Here's the drawing with two shaded views (mm, measured from the low corner). I have some questions. Give positions to 0.01 mm unless a question says otherwise; leave off trailing zeros. Loops run counter-clockwise (first coordinate to the right, second up) from the corner with the lowest first, then second, coordinate; pieces in that order, holes last. Notation, with made-up numbers: M 75.25,20 L 95.25,20 A21 ccw 95.25,39 Z; hole C 23,1.25 d8. An arc over 180 degrees is marked long. Put each result on its own line as item: value. Start each with the question number.
1) Please list where these lines run through material, in increasing order: line 1 along X through (y, z) = (25, 2.35); line 2 along Y through (x, z) = (63, 1); line 3 along X through (y, z) = (11, 2.7). Write a range as from..to.
2) Imagine slicing it at D-D (x = 92). Write out the boundary of the cut face in (y, z).
3) Imagine slicing it at C-C (z = 1). Write out the boundary of the cut face in (x, y), then the cut area to 3 significant figures.
4) Imagine slicing it at A-A (x = 57). Write out the boundary of the cut face in (y, z), then the cut area to 3 significant figures.
5) For P1, Ø1, axis at x = 22.5, y = 31.5, coming from the -Z side; P2, Ø1.5, axis at x = 50.5, z = 2, coming from the -Y side, each with a flat end and sliding along its axis, tell me the tip position at first contact or that it passes through.
6) Imagine slicing it at B-B (y = 5). Write out the boundary of the cut face in (x, z), then the cut area to 3 significant figures.
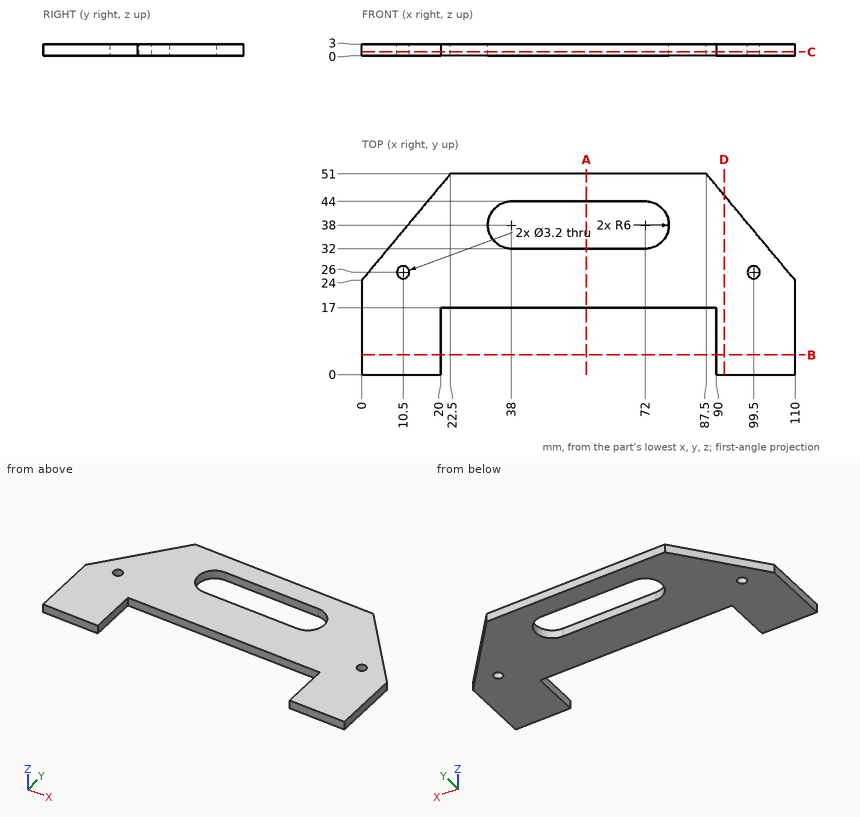
Recorded:
1. line 1: 0.83..9.25, 11.75..98.25, 100.75..109.17
1. line 2: 17..32, 44..51
1. line 3: 0..20, 90..110
2. outline: M 0,0 L 45.6,0 L 45.6,3 L 0,3 Z
3. outline: M 0,0 L 20,0 L 20,17 L 90,17 L 90,0 L 110,0 L 110,24 L 87.5,51 L 22.5,51 L 0,24 Z; hole C 10.5,26 d3.2; hole M 38,32 L 72,32 A6 ccw 72,44 L 38,44 A6 ccw Z; hole C 99.5,26 d3.2
3. area: 3,280 mm²
4. outline: M 17,0 L 32,0 L 32,3 L 17,3 Z; M 44,0 L 51,0 L 51,3 L 44,3 Z
4. area: 66.0 mm²
5. P1: z = 0
5. P2: y = 17
6. outline: M 0,0 L 20,0 L 20,3 L 0,3 Z; M 90,0 L 110,0 L 110,3 L 90,3 Z
6. area: 120 mm²
